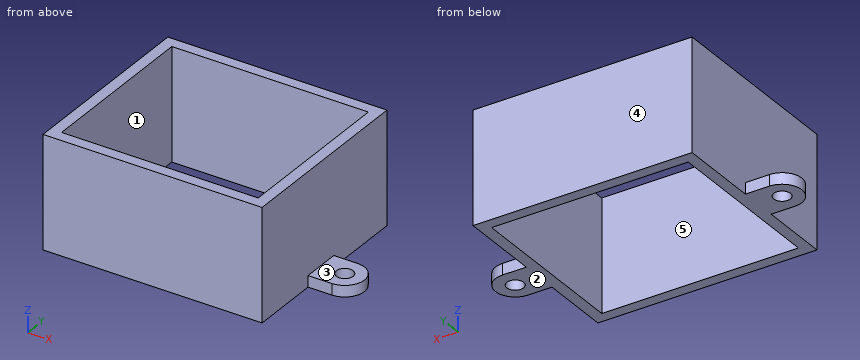
```python
from build123d import *

# Parameters (mm, degrees)
SKETCH1_W           = 35
SKETCH1_H           = 30
BOSS_EXTRUDE1_DEPTH = 20
SKETCH1_3_R         = 1.5
BOSS_EXTRUDE2_DEPTH = 2


with BuildPart() as part:
    # Sketch1 → Boss-Extrude1 (new body)
    with BuildSketch(Plane.XY):
        Polygon((37, 10.5), (37, -2), (-2, -2), (-2, 10.5), (-2, 17.5), (-2, 32), (37, 32), (37, 17.5), align=None)
        with Locations((17.5, 15)):
            Rectangle(SKETCH1_W, SKETCH1_H, mode=Mode.SUBTRACT)
    extrude(amount=BOSS_EXTRUDE1_DEPTH)

    # Sketch1_3 → Boss-Extrude2 (add)
    # profile 1 of 2: a face of its own
    with BuildSketch(Plane.XY):
        with BuildLine():
            Line((-6.25, 17.5), (-2, 17.5))
            Line((-2, 17.5), (-2, 10.5))
            Line((-2, 10.5), (-6.25, 10.5))
            ThreePointArc((-6.25, 10.5), (-9.75, 14), (-6.25, 17.5))
        make_face()
        with Locations((-6.25, 14)):
            Circle(SKETCH1_3_R, mode=Mode.SUBTRACT)
    # profile 2 of 2: a face of its own
    with BuildSketch(Plane.XY):
        with BuildLine():
            ThreePointArc((41.25, 17.5), (44.75, 14), (41.25, 10.5))
            Line((41.25, 10.5), (37, 10.5))
            Line((37, 10.5), (37, 17.5))
            Line((37, 17.5), (41.25, 17.5))
        make_face()
        with Locations((41.25, 14)):
            Circle(SKETCH1_3_R, mode=Mode.SUBTRACT)
    extrude(amount=BOSS_EXTRUDE2_DEPTH)


solid = part.part
```
Read the model definition and answer for the solid it produces. Units are mm, in the model's axes. Face numbers are marked on the shaded views. A direction names the side the tool comes from. Give positions to 0.01 mm unless a question says otherwise; leave off trailing zeros. Write each loop counter-clockwise with the first axis right and the second up, starting at its lowest first coordinate (ties: lowest second). Pieces come first, ordered by that corner, then holes. Notation, with made-up numbers: M 3.25,61 L 32.25,61 A21 cw 32.25,90 Z; hole C 27.25,53 d9. An arc over 180 degrees is marked long. Put each result on its own line as item: value. Start each with the question number.
1. The part is cut by section D-D, the plane y = 14. Give the vertices of the cut face in (x, z), and give its area (3 significant figures).
2. Consider line 1 along X through (y, z) = (21, 6.25); line 2 along Y through (x, z) = (32, 19); line 3 along Y through (x, z) = (41.25, 0.8). Determine where each line is inside the solid, lowest interval first.
3. Each of these flat-tipped pins is pushed along its axis until it touches: pin 1 Ø5.5 at (x, y) = (-4, 13.5) entering from +Z; pin 2 Ø2 at (x, z) = (-4.5, 1) entering from -Y; pin 3 Ø2 at (y, z) = (9.5, 16) entering from +X; pin 4 Ø5 at (x, y) = (41.25, 14) entering from +Z. Where does it stop, or does it pass through?
4. The part is cut by section B-B, the plane x = 29.5. Give the vertices of the cut face in (y, z).
5. For a pull along X with two mould halves and no side action, classify the marked faces 4 and 5 as released by +X, released by -X, zero draft, split by the parting line, or undercut.
6. The part is cut by section C-C, the plane z = 11.75. Give the vertices of the cut face in (x, y), and give its area (3 significant figures).
7. The part is cut by section A-A, the plane y = 19. Give the vertices of the cut face in (x, z).
8. Which of the six approach directions +Z, -Z, +X, -X, +Y, -Y give full straight-line access (tool end or side, diameter ignored) to the marked faces 1, 2 and 3?
Final values:
1. outline: M -9.75,0 L -7.75,0 L -7.75,2 L -9.75,2 Z; M -4.75,0 L 0,0 L 0,20 L -2,20 L -2,2 L -4.75,2 Z; M 35,0 L 39.75,0 L 39.75,2 L 37,2 L 37,20 L 35,20 Z; M 42.75,0 L 44.75,0 L 44.75,2 L 42.75,2 Z
1. area: 99.0 mm²
2. line 1: x = -2 to 0, 35 to 37
2. line 2: y = -2 to 0, 30 to 32
2. line 3: y = 10.5 to 12.5, 15.5 to 17.5
3. pin 1: stops at z = 20
3. pin 2: stops at y = 10.5
3. pin 3: stops at x = 37
3. pin 4: stops at z = 2
4. outline: M -2,0 L 0,0 L 0,20 L -2,20 Z; M 30,0 L 32,0 L 32,20 L 30,20 Z
5. face 4: zero draft
5. face 5: undercut
6. outline: M -2,-2 L 37,-2 L 37,32 L -2,32 Z; hole M 0,0 L 35,0 L 35,30 L 0,30 Z
6. area: 276 mm²
7. outline: M -2,0 L 0,0 L 0,20 L -2,20 Z; M 35,0 L 37,0 L 37,20 L 35,20 Z
8. face 1: +Z, -Z
8. face 2: -Z, +X, -X, +Y, -Y
8. face 3: +Z, +X, +Y, -Y
